Work out the finished part from the listing and answer in its coordinate system (mm). Face numbers are marked on the shaded views. A direction names the side the tool comes from. Round coordinates to 2 decimals unless told otherwise and drop trailing zeros. Loops run counter-clockwise (first coordinate to the right, second up) from the corner with the lowest first, then second, coordinate; pieces in that order, holes last. Notation, with made-up numbers: (84, 6) - (134, 6) arc R23 ccw to (134, 17) - close; hole circle Ø9 at (69, 3). An arc over 180 degrees is marked (long way). Use CSV: the item, a comma, the result in double quotes. Start each with the question number.
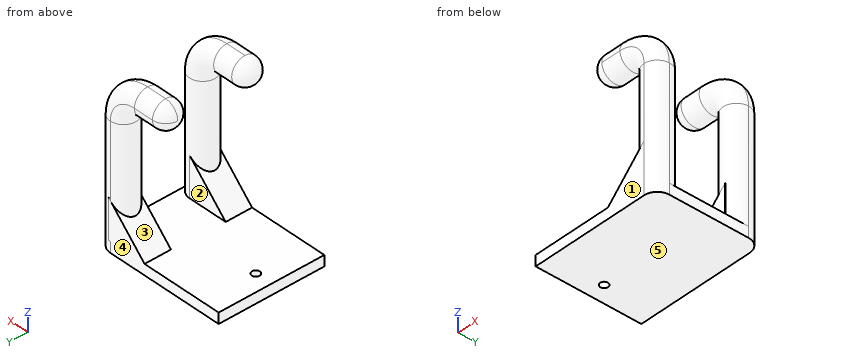
from build123d import *
from build123d import SkipClean  # not in build123d's __all__

# Parameters (mm, degrees)
F0_W      = 50
F0_H      = 40
F0_R      = 1.5
F1_DEPTH  = 4
F2_R      = 3.25
F9_R      = 5
F10_DEPTH = 2.5
F12_R     = 5
F13_DEPTH = 2.5
F14_R     = 4.9999
F17_DEPTH = 10
F18_DEPTH = 25
F20_DEPTH = 10


# Not quite as in the source:
# - a fillet or chamfer that OpenCascade refuses, or shapes differently, is made with other operations: its cross-section is extruded or revolved along the edge and cut away or added
# - a fillet or chamfer is up to 0.001 mm smaller than in the source, because OpenCascade refuses the exact size


with BuildPart() as f1:
    # F0 (on Top) → F1 (new body)
    with BuildSketch(Plane.XY):
        Rectangle(F0_W, F0_H)
        with Locations((-18.505550921, 0)):
            Circle(F0_R, mode=Mode.SUBTRACT)
    extrude(amount=F1_DEPTH)

    # F5: sweep along a path in F4
    with BuildLine(Plane.XZ.offset(-15)) as f5_path:
        Line((20, 4), (20, 46))
        ThreePointArc((20, 46), (17.0710678119, 53.0710678119), (10, 56))
        Line((10, 56), (0, 56))
    # F2 (on face) → F5 (sweep)
    with BuildSketch(Plane.XY.offset(4)):
        with BuildLine():
            ThreePointArc((20, 20), (16.4644660941, 11.4644660941), (25, 15))
            ThreePointArc((25, 15), (23.5355339059, 18.5355339059), (20, 20))
        make_face()
        with Locations((20, 15)):
            Circle(F2_R, mode=Mode.SUBTRACT)
    sweep(path=f5_path.line)

    # F8: sweep along a path in F7
    with BuildLine(Plane.XZ.offset(15)) as f8_path:
        Line((20, 4), (20, 46))
        ThreePointArc((20, 46), (17.0710678119, 53.0710678119), (10, 56))
        Line((10, 56), (0, 56))
    # F2 (on face) → F8 (sweep)
    with BuildSketch(Plane.XY.offset(4)):
        with BuildLine():
            ThreePointArc((19.9999999389, -20), (23.5355338843, -18.5355339275), (25, -15))
            ThreePointArc((25, -15), (16.4644661157, -11.4644660725), (19.9999999389, -20))
        make_face()
        with Locations((20, -15)):
            Circle(F2_R, mode=Mode.SUBTRACT)
    sweep(path=f8_path.line)

    # F9 (on face) → F10 (join)
    with BuildSketch(Plane(origin=(0, 0, 0), x_dir=(0, -1, 0), z_dir=(-1, 0, 0))):
        with Locations((15, 56)):
            Circle(F9_R)
    extrude(amount=F10_DEPTH)

    # F11: fillet of radius 5 on 1 edges, made by hand

    # F11_s1 → F11_t2 (revolve, cut)
    with BuildSketch(Plane.XY.offset(56)):
        with BuildLine():
            ThreePointArc((2.5, -20), (-1.0355339059, -18.5355339059), (-2.5, -15))
            Line((-2.5, -15), (-2.5, -20))
            Line((-2.5, -20), (2.5, -20))
        make_face()
    revolve(axis=Axis((-2.5, -15, 56), (-1, 0, 0)), mode=Mode.SUBTRACT)

    # F12 (on face) → F13 (join)
    with BuildSketch(Plane(origin=(0, 0, 0), x_dir=(0, -1, 0), z_dir=(-1, 0, 0))):
        with Locations((-15, 56)):
            Circle(F12_R)
    extrude(amount=F13_DEPTH)

    # F14 (radius 5 in the source; OpenCascade refuses exactly that, so slightly less here)
    f14_edges = [f1.edges().sort_by_distance(p)[0] for p in [
        (-2.5, 20, 56),
        (25, 20, 2),
        (25, -20, 2),
    ]]
    fillet(f14_edges, radius=F14_R)

    # F16 (on offset) → F17 (join)
    with BuildSketch(Plane(origin=(0, 10, 0), x_dir=(-1, 0, 0), z_dir=(0, 1, 0))):
        Polygon((-20.7827799022, 4), (-5.7827799022, 4), (-20.7827799022, 19), align=None)
    with SkipClean():  # cleaning this boolean's faces spoils the solid; the shape is the same uncleaned
        extrude(amount=F17_DEPTH)

    # F2 (on face) → F18 (cut)
    with BuildSketch(Plane.XY.offset(4)):
        with BuildLine():
            Line((25, -20), (25, -15))
            ThreePointArc((25, -15), (23.5355338843, -18.5355339275), (19.9999999389, -20))
            Line((19.9999999389, -20), (25, -20))
        make_face()
        with BuildLine():
            ThreePointArc((20, 20), (23.5355339059, 18.5355339059), (25, 15))
            Line((25, 15), (25, 20))
            Line((25, 20), (20, 20))
        make_face()
    extrude(amount=-F18_DEPTH, mode=Mode.SUBTRACT)

    # F19 (on face) → F20 (join)
    with BuildSketch(Plane.XZ.offset(20)):
        Polygon((5, 4), (20, 4), (20, 19), align=None)
    extrude(amount=-F20_DEPTH)


solid = f1.part
Item 1: The mould has two halves that part along Z. Classify the marked faces 3, 4 and 5: pulls with the +Z half, pulls with the -Z half, needs draft (parallel to the pull), parting line crosses it, or undercut.
Item 2: Find the intervals of material crossed by probe 1 along Y at (x, z) = (5, 56); probe 2 along Z at (x, y) = (3, -15); probe 3 along Z at (x, y) = (0.5, 14), in increasing order. Write a range as [from, to].
Item 3: Which of the six approach directions +Z, -Z, +X, -X, +Y, -Y give full straight-line access (tool end or side, diameter ignored) to the marked faces 1 and 2?
Item 4: A cutting plane is placed at A-A (z = 30.5). Determine the outline of the cut face in (x, y), plus the area to 3 significant figures.
Item 5: Each of these flat-tipped pins is pushed along its axis until it touches: pin 1 Ø3 at (y, z) = (-15.5, 56.5) entering from +X; pin 2 Ø1.5 at (y, z) = (-16, 32) entering from +X; pin 3 Ø10 at (y, z) = (8.5, 25.5) entering from -X; pin 4 Ø2.5 at (x, y) = (-18.51, 0) entering from +Z. Where does it stop, or does it pass through?
Item 6: A cutting plane is placed at B-B (y = -11). Determine the outline of the cut face in (x, z).
Item 7: A cutting plane is placed at C-C (x = 1). State how many separate pieces and enclosed holes the cut face has, plus the area to 3 significant figures.
Item 8: A cutting plane is placed at D-D (x = -12). Determine the outline of the cut face in (y, z), plus the area to 3 significant figures.
Result sheet:
1,face 3,"undercut"
1,face 4,"needs draft"
1,face 5,"pulls with the -Z half"
2,probe 1,"[-20, -18.25], [-11.75, -10], [10, 11.75], [18.25, 20]"
2,probe 2,"[0, 4], [51, 52.75], [59.25, 61]"
2,probe 3,"[0, 4], [51.53, 52.91], [59.09, 60.47]"
3,face 1,"+Z, -Z, +X, -X, -Y"
3,face 2,"+Z, +X, -X"
4,outline,"circle Ø10 at (20, -15); circle Ø10 at (20, 15); hole circle Ø6.5 at (20, -15); hole circle Ø6.5 at (20, 15)"
4,area,"90.7 mm^2"
5,pin 1,"x = 21.98"
5,pin 2,"x = 24.99"
5,pin 3,"x = 15.23"
5,pin 4,"through"
6,outline,"(-25, 0) - (25, 0) - (25, 4) - (23, 4) - (23, 46) arc R13 ccw to (10, 59) - (2.5, 59) arc R3 ccw to (2.5, 53) - (10, 53) arc R7 cw to (17, 46) - (17, 16) - (5, 4) - (-25, 4) - close"
7,separate pieces,"3"
7,enclosed holes,"2"
7,area,"237 mm^2"
8,outline,"(-20, 0) - (20, 0) - (20, 4) - (-20, 4) - close"
8,area,"160 mm^2"
